from build123d import *

# Parameters (mm, degrees)
F0_W     = 330.2
F0_H     = 762
F0_W_2   = 203.2
F0_H_2   = 635
F1_DEPTH = 374.65
F2_DEPTH = 6.35
F3_W     = 374.65
F3_H     = 762
F3_W_2   = 247.65
F3_H_2   = 635
F4_DEPTH = 19.05
F5_DEPTH = 12.7


# Not quite as in the source:
# - a feature names something its author has since deleted; it is built from what else it names


with BuildPart() as f1:
    # F0 (on Front) → F1 (new body)
    with BuildSketch(Plane.XZ):
        with Locations((48.0267770052, 381)):
            Rectangle(F0_W, F0_H)
        with Locations((48.0267770052, 381)):
            Rectangle(F0_W_2, F0_H_2, mode=Mode.SUBTRACT)
        with Locations((48.0267770052, 381)):
            Rectangle(F0_W_2, F0_H_2)
    extrude(amount=-F1_DEPTH)

    # F0 (on Front) → F2 (cut)
    with BuildSketch(Plane.XZ):
        with Locations((48.0267770052, 381)):
            Rectangle(F0_W_2, F0_H_2)
    extrude(amount=-F2_DEPTH, mode=Mode.SUBTRACT)

    # F3 (on face) → F4 (join)
    with BuildSketch(Plane.YZ.offset(213.1267770052)):
        with Locations((187.325, 381)):
            Rectangle(F3_W, F3_H)
        with Locations((187.325, 381)):
            Rectangle(F3_W_2, F3_H_2, mode=Mode.SUBTRACT)
    extrude(amount=F4_DEPTH)

    # F5 (add): a face of the model
    f5_faces = [f1.faces().sort_by_distance(p)[0] for p in [
        (213.1267770052, 187.325, 381),
    ]]
    extrude(f5_faces, amount=F5_DEPTH)


solid = f1.part
CAD build for the part. Positions are in the model's coordinates, mm. A direction names the side the tool comes from. Round coordinates to 2 decimals unless told otherwise and drop trailing zeros. Write each loop counter-clockwise with the first axis right and the second up, starting at its lowest first coordinate (ties: lowest second). Pieces come first, ordered by that corner, then holes. Notation, with made-up numbers: (6, 20) -> (24, 20) arc R23 cw to (24, 51) -> close; hole circle Ø7 at (50.25, -33.75). An arc over 180 degrees is marked (long way). Answer as a JSON object with one key per item and string values.
(1) Pin check, flat tips, straight feed: P1, Ø1, axis at y = 300, z = 393.5, coming from the +X side; P2, Ø1.5, axis at x = -50, z = 480.5, coming from the -Y side. Stop position of each tip, or through.
Reported:
{"P1": "stops at x = 225.83", "P2": "stops at y = 6.35"}
(2) Probe probe 1 along Y at (x, z) = (96, 410); probe 2 along X at (y, z) = (261, 250.5). List the from-to ranges inside material, lowest first. Write a range as [from, to].
Reported:
{"probe 1": "y = [6.35, 374.65]", "probe 2": "x = [-117.07, 225.83]"}
(3) Which spindle directions (+Z, -Z, +X, -X, +Y, -Y) get a long thin tool onto all of the face, cutting with end or side? Do faces 4 (the face through (47, 6.35, 385)), 5 (the face through (232.177, 60, 386)). Say none if no direction does.
Reported:
{"face 4": "-Y", "face 5": "+Z, -Z, +X, +Y, -Y"}
(4) Two-plate mould, pull along Z, no slides. Class faces 1 (the face through (225.827, 186, 377)), 2 (the face through (55, 185, 762)), 3 (the face through (-117.073, 185, 376)): +Z half, -Z half, draft (parallel to the pull), parting line (faces both ways), or undercut.
Reported:
{"face 1": "undercut", "face 2": "+Z half", "face 3": "draft"}
(5) Band-saw the part on B-B, the plane z = 337.5. List the corners of the cut face in (x, y), then the cut area to 3 significant figures.
Reported:
{"outline": "(-117.07, 0) -> (-53.57, 0) -> (-53.57, 6.35) -> (149.63, 6.35) -> (149.63, 0) -> (232.18, 0) -> (232.18, 63.5) -> (225.83, 63.5) -> (225.83, 311.15) -> (232.18, 311.15) -> (232.18, 374.65) -> (-117.07, 374.65) -> close", "area": "128,000 mm^2"}
(6) Band-saw the part on A-A, the plane y = 135. List the corners of the cut face in (x, z).
Reported:
{"outline": "(-117.07, 0) -> (232.18, 0) -> (232.18, 63.5) -> (225.83, 63.5) -> (225.83, 698.5) -> (232.18, 698.5) -> (232.18, 762) -> (-117.07, 762) -> close"}
